Read the model definition and answer for the solid it produces. Units are mm, in the model's axes. A direction names the side the tool comes from. Coordinates: 2 decimals unless noted, no trailing zeros. Write each loop counter-clockwise with the first axis right and the second up, starting at its lowest first coordinate (ties: lowest second). Pieces come first, ordered by that corner, then holes. Notation, with made-up numbers: M 61,59 L 108,59 A22 ccw 108,81 Z; hole C 33.25,-18 d3. An arc over 180 degrees is marked long. Use a Markdown table: item, result. Add a question column.
from build123d import *

# Parameters (mm, degrees)
F1_DEPTH = 71
F3_D     = 3.2
F3_DEPTH = 14.85
F3_TIP   = 0.9613769904


with BuildPart() as f1:
    # F0 (on Front) → F1 (new body)
    with BuildSketch(Plane.XZ):
        with BuildLine():
            Line((22.000012, -13.4738130626), (22.000012, 0.9761649373))
            Line((22.000012, 0.9761649373), (22.000012, 9.6261749373))
            Line((22.000012, 9.6261749373), (20.950012, 10.6761749374))
            Line((20.950012, 10.6761749374), (12.049988, 10.6761749373))
            Line((12.049988, 10.6761749373), (11.549988, 10.1761749373))
            Line((11.549988, 10.1761749373), (5.2, 10.1761749373))
            Line((5.2, 10.1761749373), (4.7, 10.6761749373))
            Line((4.7, 10.6761749373), (-4.7, 10.6761749373))
            Line((-4.7, 10.6761749373), (-5.2, 10.1761749373))
            Line((-5.2, 10.1761749373), (-11.549988, 10.1761749373))
            Line((-11.549988, 10.1761749373), (-12.049988, 10.6761749373))
            Line((-12.049988, 10.6761749373), (-20.950012, 10.6761749373))
            Line((-20.950012, 10.6761749373), (-22.000012, 9.6261749373))
            Line((-22.000012, 9.6261749373), (-22.000012, 0.9761649373))
            Line((-22.000012, 0.9761649373), (-22.000012, -13.4738130627))
            Line((-22.000012, -13.4738130627), (-20.75, -14.7238250627))
            Line((-20.75, -14.7238250627), (-9.5804297104, -14.7238250627))
            Line((-9.5804297104, -14.7238250627), (-7.8, -12.601991559))
            Line((-7.8, -12.601991559), (-7.8, -8.2738250627))
            Line((-7.8, -8.2738250627), (-8.502817534, -7.5710075287))
            ThreePointArc((-8.502817534, -7.5710075287), (-8.962563133, -6.7863881956), (-9.7471824661, -6.3266425966))
            Line((-9.7471824661, -6.3266425966), (-10, -6.0738250627))
            Line((-10, -6.0738250627), (-10, -4.5738250627))
            Line((-10, -4.5738250627), (-9.747182466, -4.3210075287))
            ThreePointArc((-9.747182466, -4.3210075287), (-8.962563133, -3.8612619297), (-8.502817534, -3.0766425966))
            Line((-8.502817534, -3.0766425966), (-8.25, -2.8238250627))
            Line((-8.25, -2.8238250627), (8.25, -2.8238250628))
            Line((8.25, -2.8238250628), (8.502817534, -3.0766425968))
            ThreePointArc((8.502817534, -3.0766425968), (8.9625631329, -3.8612619298), (9.747182466, -4.3210075287))
            Line((9.747182466, -4.3210075287), (10, -4.5738250627))
            Line((10, -4.5738250627), (10, -6.0738250627))
            Line((10, -6.0738250627), (9.747182466, -6.3266425966))
            ThreePointArc((9.747182466, -6.3266425966), (8.9625631329, -6.7863881956), (8.5028175339, -7.5710075287))
            Line((8.5028175339, -7.5710075287), (7.8, -8.2738250627))
            Line((7.8, -8.2738250627), (7.8, -12.601991559))
            Line((7.8, -12.601991559), (9.5804297104, -14.7238250627))
            Line((9.5804297104, -14.7238250627), (20.75, -14.7238250627))
            Line((20.75, -14.7238250627), (22.000012, -13.4738130626))
        make_face()
    extrude(amount=F1_DEPTH)

    # F3
    with Locations(Plane.XY.offset(10.6761749373)):
        with Locations((-16, -17.5), (-16, -53.5), (16, -53.5), (16, -17.5)):
            Hole(F3_D / 2, depth=F3_DEPTH)
            with Locations((0, 0, -(F3_DEPTH + F3_TIP / 2))):  # 118° drill point
                Cone(0, F3_D / 2, F3_TIP, mode=Mode.SUBTRACT)


solid = f1.part
Item 1: Find section A-A on x = 4. Give the vertices of the cut face in (y, z), then the cut area to 4 significant figures.
Item 2: For faces 1 (the flat face through (8, -35, 10.176)), 2 (the flat face through (8.68, -35, -13.65)), 3 (the flat face through (-15, -35, -14.724)), determine the directions among +Z, -Z, +X, -X, +Y, -Y from which every point of the face is accessible in a straight line to the end or side of a thin tool.
Item 3: Each of these flat-tipped pins is pushed along its axis until it touches: pin 1 (10 mm diameter, centred on x = 8, y = -9, fed in from +Z); pin 2 (1.9 mm diameter, centred on x = 16, y = -17.5, fed in from +Z); pin 3 (13 mm diameter, centred on x = 2, y = -51, fed in from -Z); pin 4 (3 mm diameter, centred on x = -9.5, y = -36.5, fed in from +Z). Where does it stop, or does it pass through?
Item 4: Find section B-B on x = -6. Give the vertices of the cut face in (y, z), then the cut area to 3 significant figures.
Item 5: Consider probe 1 along X at (y, z) = (-53.5, 6.25); probe 2 along Y at (x, z) = (16, 4.75); probe 3 along X at (y, z) = (-16, -9.5). Determine where each line is inside the solid, lowest interval first.
Item 6: Determine the mould class of faces 4 (the cylindrical face through (-14.4, -53.43, 3.15)), 5 (the conical face through (16.257, -53.606, -4.968)), 6 (the flat face through (10, -35, -5)) for opening direction Z: pulls with the +Z half, pulls with the -Z half, needs draft (parallel to the pull), parting line crosses it, or undercut.
Geometry says:
| question | item | result |
|---|---|---|
| 1 | outline | M -71,-2.82 L 0,-2.82 L 0,10.68 L -71,10.68 Z |
| 1 | area | 958.5 mm2 |
| 2 | face 1 | +Z, +Y, -Y |
| 2 | face 2 | -Z, +Y, -Y |
| 2 | face 3 | -Z, +X, -X, +Y, -Y |
| 3 | pin 1 | stops at z = 10.68 |
| 3 | pin 2 | stops at z = -4.56 |
| 3 | pin 3 | stops at z = -13.44 |
| 3 | pin 4 | stops at z = 10.18 |
| 4 | outline | M -71,-2.82 L 0,-2.82 L 0,10.18 L -71,10.18 Z |
| 4 | area | 923 mm2 |
| 5 | probe 1 | x = -22 to -17.6, -14.4 to 14.4, 17.6 to 22 |
| 5 | probe 2 | y = -71 to -55.1, -51.9 to -19.1, -15.9 to 0 |
| 5 | probe 3 | x = -22 to -7.8, 7.8 to 22 |
| 6 | face 4 | needs draft |
| 6 | face 5 | pulls with the +Z half |
| 6 | face 6 | undercut |
